For this review, take the finished solid that the model builds, in its own axes (mm). A direction names the side the tool comes from. Give positions to 0.01 mm unless a question says otherwise; leave off trailing zeros. Write each loop counter-clockwise with the first axis right and the second up, starting at its lowest first coordinate (ties: lowest second). Pieces come first, ordered by that corner, then holes. Notation, with made-up numbers: M 8,-11 L 59,-11 A23 cw 59,1 Z; hole C 87,23 d9. An arc over 180 degrees is marked long. Write item = value, one per line.
```python
from build123d import *

# Parameters (mm, degrees)
EXTRUDE_THIN1_DEPTH = 571.5
FILLET1_R           = 1.016


with BuildPart() as part:
    # Sketch1 → Extrude-Thin1 (new body)
    with BuildSketch(Plane.XY):
        with BuildLine():
            Line((0, 0), (-2.38125, 0))
            ThreePointArc((-2.38125, 0), (-3.372303364, 3.783352795), (-6.090912463, 6.59495549))
            ThreePointArc((-6.090912463, 6.59495549), (-8.607567743, 9.197696269), (-9.525, 12.7))
            Line((-9.525, 12.7), (-11.1125, 12.7))
            Line((-11.1125, 12.7), (-11.1125, 49.2125))
            ThreePointArc((-11.1125, 49.2125), (-11.577467985, 50.335032015), (-12.7, 50.8))
            Line((-12.7, 50.8), (-12.7, 57.15))
            Line((-12.7, 57.15), (1.5875, 57.15))
            Line((1.5875, 57.15), (1.5875, 56.134))
            Line((1.5875, 56.134), (-11.684, 56.134))
            Line((-11.684, 56.134), (-11.684, 51.609572433))
            ThreePointArc((-11.684, 51.609572433), (-10.529358591, 50.650042391), (-10.0965, 49.2125))
            Line((-10.0965, 49.2125), (-10.0965, 13.716))
            Line((-10.0965, 13.716), (-8.424185054, 13.716))
            ThreePointArc((-8.424185054, 13.716), (-7.953453255, 10.150515553), (-5.563316024, 7.463228487))
            ThreePointArc((-5.563316024, 7.463228487), (-2.749191769, 4.717697591), (-1.424552135, 1.016))
            Line((-1.424552135, 1.016), (0, 1.016))
            Line((0, 1.016), (0, 0))
        make_face()
    extrude(amount=-EXTRUDE_THIN1_DEPTH)

    # Fillet1
    fillet1_edges = [part.edges().sort_by_distance(p)[0] for p in [
        (-8.424185054, 13.716, -285.75),
        (-2.38125, 0, -285.75),
        (-11.1125, 12.7, -285.75),
        (-12.7, 50.8, -285.75),
        (-12.7, 57.15, -285.75),
    ]]
    fillet(fillet1_edges, radius=FILLET1_R)


solid = part.part
```
1. Machinability: for faces 1 (the face through (-10.3, 37.2, 0)), 2 (the face through (-5, 56.134, -282)), which of the approach directions +Z, -Z, +X, -X, +Y, -Y give a long, thin tool a straight path to every point of the face, cutting with its end or side? Answer none if there is none.
Responses:
face_1 = +Z, +X, -X, +Y, -Y
face_2 = +Z, -Z, +X
2. The part is to be moulded in two halves that separate along Y. For faces 3 (the face through (-10.096, 32, -282)), 4 (the face through (-5, 57.15, -282)), 5 (the face through (-11.112, 31, -282)), say which applies: +Y half, -Y half, draft (parallel to the pull), parting line (faces both ways), or undercut.
Responses:
face_3 = undercut
face_4 = +Y half
face_5 = draft
3. Insertion check: P1, Ø1, axis at y = 15, z = -389.5, coming from the -X side; P2, Ø3.5, axis at y = 54, z = -375.5, coming from the +X side; P3, Ø1.5, axis at y = 8.5, z = -407, coming from the +X side. Each pin has a flat end and moves straight along its axis. Give the tip position at first contact, or say it passes through.
Responses:
P1 = -11.11
P2 = -11.68
P3 = -5.99
4. For line 1 along X through (y, z) = (37, -341); line 2 along Y through (x, z) = (-4.5, -81); line 3 along Y through (x, z) = (0.25, -387), list the stretches that pass through material, from the lowest coordinate up. Write a range as from..to.
Responses:
line_1 = -11.11..-10.1
line_2 = 5.31..6.7, 56.13..57.15
line_3 = 56.13..57.15
5. We need section B-B, the plane y = 37.5. Write out the cut boundary in (x, z).
Responses:
outline = M -11.11,-571.5 L -10.1,-571.5 L -10.1,0 L -11.11,0 Z
